Part model, mm, in its own coordinate system. A direction names the side the tool comes from. Round coordinates to 2 decimals unless told otherwise and drop trailing zeros. Loops run counter-clockwise (first coordinate to the right, second up) from the corner with the lowest first, then second, coordinate; pieces in that order, holes last.
(1) Probe probe 1 along Z at (x, y) = (10, 3.5); probe 2 along X at (y, z) = (12.5, -5); probe 3 along Z at (x, y) = (5.5, 6.75). List the from-to ranges inside material, lowest first.
(2) Flat gauge pins, fed straight in: pin 1 (9.5 mm diameter, centred on x = 10, z = -10, fed in from +Y); pin 2 (6.5 mm diameter, centred on x = 11, z = -18.5, fed in from +Y); pin 3 (12 mm diameter, centred on x = 11, y = 13.5, fed in from -Z). Where does each tip first touch, or does it go through?
(3) Cut at A-A on y = 16. List the corners of the cut face in (x, z), then the cut area to 3 significant figures.
(4) Cut at B-B on x = 5.5. List the corners of the cut face in (y, z), then the cut area to 4 significant figures.
(5) Tool access for faces 5 (the face through (7.5, 15, -1)), 6 (the face through (10, 3, -19)), 7 (the face through (7, 13, -2)): list every direction of +Z, -Z, +X, -X, +Y, -Y with a clear straight run to the whole face (end or side of a thin tool).
(6) Cut at C-C on z = -6. List the corners of the cut face in (x, y), then the cut area to 3 significant figures.
(7) Cut at D-D on x = 3.5. List the corners of the cut face in (y, z), then the cut area to 3 significant figures.
(8) Mould opens along X. For faces 1 (the face through (20, 10, -12)), 2 (the face through (10.16, 5, -13.34)), 3 (the face through (10, 3, -25)), 4 (the face through (5.598, 13.244, -1.014)) say: +X half, -X half, draft (parallel to the pull), parting line (faces both ways), or undercut.
from build123d import *

# Parameters (mm, degrees)
IZIM1_W                     = 20
IZIM1_H                     = 25
Y_KSEKLIK_EKSTR_ZYON1_DEPTH = 20
KES_EKSTR_ZYON3_DEPTH       = 32
IZIM3_R                     = 3
KES_EKSTR_ZYON4_DEPTH       = 17
Y_KSEKLIK_EKSTR_ZYON2_DEPTH = 2
IZIM5_R                     = 0.75
KES_EKSTR_ZYON5_DEPTH       = 32


with BuildPart() as part:
    # Çizim1 → Yükseklik-Ekstrüzyon1 (new body)
    with BuildSketch(Plane(origin=(0, 0, 0), x_dir=(1, 0, 0), z_dir=(0, 1, 0))):
        with Locations((10, 12.5)):
            Rectangle(IZIM1_W, IZIM1_H)
    extrude(amount=Y_KSEKLIK_EKSTR_ZYON1_DEPTH)

    # Çizim2 → Kes-Ekstrüzyon3 (cut)
    with BuildSketch(Plane.XY):
        with BuildLine():
            Line((2.5, 12.5), (2.5, 20))
            Line((2.5, 20), (17.5, 20))
            Line((17.5, 20), (17.5, 12.5))
            ThreePointArc((17.5, 12.5), (10, 5), (2.5, 12.5))
        make_face()
    extrude(amount=-KES_EKSTR_ZYON3_DEPTH, mode=Mode.SUBTRACT)

    # Çizim3 → Kes-Ekstrüzyon4 (cut)
    with BuildSketch(Plane(origin=(0, 20, 0), x_dir=(1, 0, 0), z_dir=(0, 1, 0))):
        with Locations(Location((10, 10, 0), (0, 0, 270))):
            Circle(IZIM3_R)
        with Locations(Location((10, 19, 0), (0, 0, 270))):
            Circle(IZIM3_R)
    extrude(amount=-KES_EKSTR_ZYON4_DEPTH, mode=Mode.SUBTRACT)

    # Çizim4 → Yükseklik-Ekstrüzyon2 (add)
    with BuildSketch(Plane.XY):
        Polygon((12.5, 20), (20, 20), (20, 0), (0, 0), (0, 20), (7.5, 20), (7.5, 10), (12.5, 10), align=None)
    extrude(amount=-Y_KSEKLIK_EKSTR_ZYON2_DEPTH)

    # Çizim5 → Kes-Ekstrüzyon5 (cut)
    with BuildSketch(Plane(origin=(0, 0, -25), x_dir=(-1, 0, 0), z_dir=(0, 0, -1))):
        with Locations((-14.5, 12.5)):
            Circle(IZIM5_R)
        with Locations((-5.5, 12.5)):
            Circle(IZIM5_R)
    extrude(amount=-KES_EKSTR_ZYON5_DEPTH, mode=Mode.SUBTRACT)


solid = part.part
Final values:
1. probe 1: z = -25 to -22, -16 to -13, -7 to 0
1. probe 2: x = 0 to 2.5, 17.5 to 20
1. probe 3: z = -2 to 0
2. pin 1: stops at y = 6.7
2. pin 2: stops at y = 6.32
2. pin 3: stops at z = -2
3. outline: (0, -25) - (2.5, -25) - (2.5, -2) - (7.5, -2) - (7.5, 0) - (0, 0) - close; (12.5, -2) - (17.5, -2) - (17.5, -25) - (20, -25) - (20, 0) - (12.5, 0) - close
3. area: 145 mm2
4. outline: (0, -25) - (6.5, -25) - (6.5, -2) - (11.75, -2) - (11.75, 0) - (0, 0) - close; (13.25, -2) - (20, -2) - (20, 0) - (13.25, 0) - close
4. area: 186.5 mm2
5. face 5: +Z, -Z, +Y
5. face 6: +Y
5. face 7: -Z, +Y
6. outline: (0, 0) - (20, 0) - (20, 20) - (17.5, 20) - (17.5, 12.5) arc R7.5 cw to (2.5, 12.5) - (2.5, 20) - (0, 20) - close
6. area: 199 mm2
7. outline: (0, -25) - (8.76, -25) - (8.76, -2) - (20, -2) - (20, 0) - (0, 0) - close
7. area: 241 mm2
8. face 1: +X half
8. face 2: undercut
8. face 3: draft
8. face 4: undercut
